Check sheet for the modelled part. Datum: model origin and axes. Units: mm. Face numbers are marked on the shaded views. A direction names the side the tool comes from. Give positions to 0.01 mm unless a question says otherwise; leave off trailing zeros. Write each loop counter-clockwise with the first axis right and the second up, starting at its lowest first coordinate (ties: lowest second). Pieces come first, ordered by that corner, then holes. Notation, with made-up numbers: M -31,63 L 10,63 A25 ccw 10,75 Z; hole C -5.75,72 d8. An arc over 180 degrees is marked long. Write item = value, one per line. Start each with the question number.
1) Sectioned sample at B-B, the plane x = -0.25. Record the cut outline in (y, z).
2) Sectioned sample at D-D, the plane y = -7.25. Record the cut outline in (x, z), then the cut area to 3 significant figures.
3) Gauge pin test, flat end, axial feed: pin 1 (1.5 mm diameter, centred on x = -0.5, y = -10.5, fed in from +Z). Record the tip position at first contact, or that the pin passes through.
4) Scan lines: L1, parallel to Y at x = 2.75, z = 1.25; L2, parallel to Z at x = 2.5, y = -8.5; L3, parallel to X at y = -1.75, z = 1.6. Record each from-to range of solid material in increasing order.
5) Sectioned sample at A-A, the plane z = 1.6. Record the cut outline in (x, y), then the cut area to 3 significant figures.
6) Sectioned sample at C-C, the plane x = 4.25. Record the cut outline in (y, z) (3 decimals), then the cut area to 3 significant figures.
7) Set-up check for the marked faces 1 and 2: record each of +Z, -Z, +X, -X, +Y, -Y from which the full face is reachable in a straight line by a thin tool's end or side.
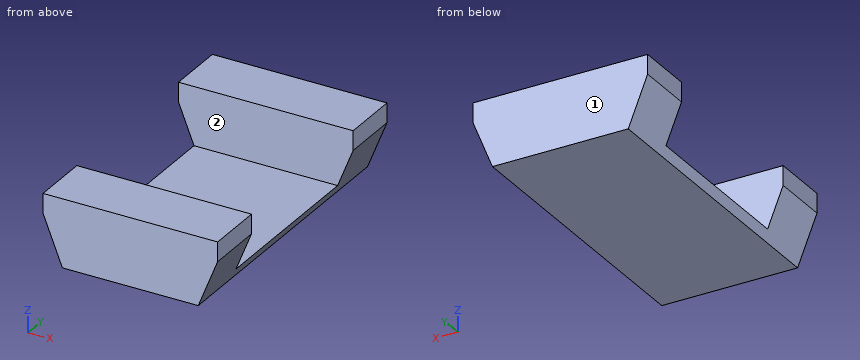
from build123d import *

# Parameters (mm, degrees)
F1_DEPTH = 15
F3_DEPTH = 3


with BuildPart() as f1:
    # F0 (on Front) → F1 (new body)
    with BuildSketch(Plane.XZ):
        Polygon((-3.5, 0), (0, 0), (3.5, 0), (4.5, 2.5), (4.5, 3.5), (0, 3.5), (-4.5, 3.5), (-4.5, 2.5), align=None)
    extrude(amount=F1_DEPTH)

    # F2 (on face) → F3 (cut)
    with BuildSketch(Plane.XY.offset(3.5)):
        Polygon((4.5, -12), (4.5, -7.5), (4.5, -3), (-4.5, -3), (-4.5, -7.5), (-4.5, -12), align=None)
    extrude(amount=-F3_DEPTH, mode=Mode.SUBTRACT)


solid = f1.part
Data:
q1.outline = M -15,0 L 0,0 L 0,3.5 L -3,3.5 L -3,0.5 L -12,0.5 L -12,3.5 L -15,3.5 Z
q2.outline = M -3.7,0.5 L -3.5,0 L 3.5,0 L 3.7,0.5 Z
q2.area = 3.60 mm2
q3.pin_1 = 0.5
q4.L1 = -15 to -12, -3 to 0
q4.L2 = 0 to 0.5
q4.L3 = -4.14 to 4.14
q5.outline = M -4.14,-15 L 4.14,-15 L 4.14,-12 L -4.14,-12 Z; M -4.14,-3 L 4.14,-3 L 4.14,0 L -4.14,0 Z
q5.area = 49.7 mm2
q6.outline = M -15,1.875 L -12,1.875 L -12,3.5 L -15,3.5 Z; M -3,1.875 L 0,1.875 L 0,3.5 L -3,3.5 Z
q6.area = 9.75 mm2
q7.face_1 = +Z, -Z, +X, -X, +Y
q7.face_2 = +Z, +X, -X
